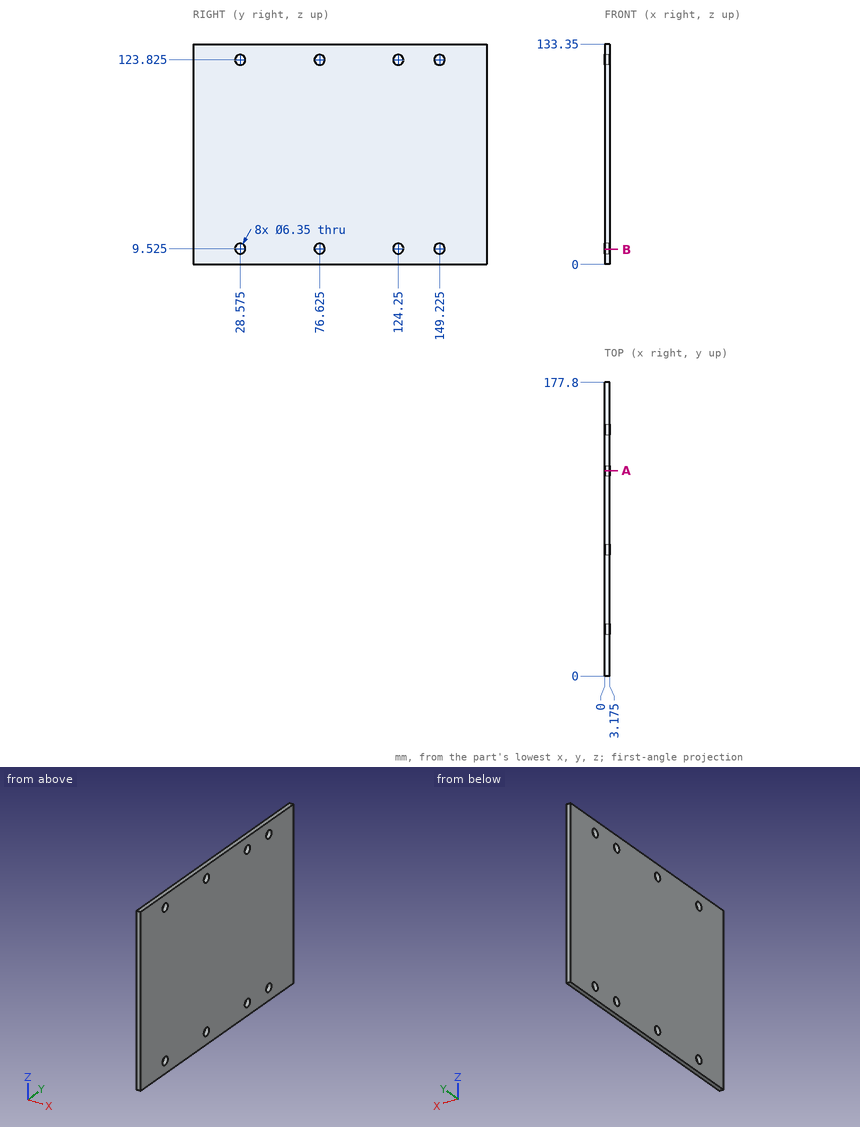
The figure shows three views and two pictorial views of one solid part (mm, origin at its lowest corner). Answer the questions. Give positions to 0.01 mm unless a question says otherwise; leave off trailing zeros. Order: outer loops, then holes, each group sorted by start corner. A loop starts at its lowest first (then second) coordinate and runs counter-clockwise, first axis right, second up. Notation, with made-up numbers: (-37.75, -21) -> (6.25, -21) arc R16 ccw to (6.25, 6) -> close; hole circle Ø5 at (-10.75, -39.5). An arc over 180 degrees is marked (long way). Answer as a JSON object with one key per item and string values. Group by question number.
Item 1: Consider L1, parallel to Z at x = 0.9, y = 124.25; L2, parallel to Y at x = 0.6, z = 121.5; L3, parallel to Z at x = 1.3, y = 79. Determine where each line is inside the solid, lowest interval first. Write a range as from..to.
Item 2: A flat-ended cylindrical pin translates along its axis: pin 1 (5 mm diameter, centred on y = 149.225, z = 9.525, fed in from +X). Find the tip coordinate at first contact, or state that the pin passes through.
Item 3: The part is cut by section B-B on z = 9. Write down the section's boundary in (x, y) (3 decimals), and give its area (3 significant figures).
Item 4: The part is cut by section A-A on y = 124.25. Write down the section's boundary in (x, z) (3 decimals), and give its area (3 significant figures).
Result set:
{
 "1": {"L1": "0..6.35, 12.7..120.65, 127..133.35", "L2": "0..26.41, 30.74..74.46, 78.79..122.09, 126.41..147.06, 151.39..177.8", "L3": "0..7.42, 11.63..121.72, 125.93..133.35"},
 "2": {"pin 1": "through"},
 "3": {"outline": "(0, 0) -> (3.175, 0) -> (3.175, 25.444) -> (0, 25.444) -> close; (0, 31.706) -> (3.175, 31.706) -> (3.175, 73.494) -> (0, 73.494) -> close; (0, 79.756) -> (3.175, 79.756) -> (3.175, 121.119) -> (0, 121.119) -> close; (0, 127.381) -> (3.175, 127.381) -> (3.175, 146.094) -> (0, 146.094) -> close; (0, 152.356) -> (3.175, 152.356) -> (3.175, 177.8) -> (0, 177.8) -> close", "area": "485 mm²"},
 "4": {"outline": "(0, 0) -> (3.175, 0) -> (3.175, 6.35) -> (0, 6.35) -> close; (0, 12.7) -> (3.175, 12.7) -> (3.175, 120.65) -> (0, 120.65) -> close; (0, 127) -> (3.175, 127) -> (3.175, 133.35) -> (0, 133.35) -> close", "area": "383 mm²"}
}
